```python
from build123d import *

# Parameters (mm, degrees)
EXTRUSION1_DEPTH                  = 3
ESQUISSE2_W                       = 3
ESQUISSE2_H                       = 3
EXTRUSION2_DEPTH                  = 1.2
ESQUISSE3_W                       = 3
ESQUISSE3_H                       = 3
EXTRUSION3_DEPTH                  = 1.2
DIAM_TRE_DU_PER_AGE_4_0_4_1_D     = 4
DIAM_TRE_DU_PER_AGE_4_0_4_1_DEPTH = 3
DIAM_TRE_DU_PER_AGE_4_0_4_1_TIP   = 1.201721238


with BuildPart() as part:
    # Esquisse1 → Extrusion1 (new body, symmetric)
    with BuildSketch(Plane.XY):
        with BuildLine():
            Line((0, 0), (0, 1.5))
            ThreePointArc((0, 1.5), (3.484063784, 6.45860997), (8, 10.5))
            Line((8, 10.5), (30, 10.5))
            Line((30, 10.5), (30, -0.2))
            Line((30, -0.2), (27, -0.2))
            Line((27, -0.2), (27, 3.5))
            Line((27, 3.5), (14, 3.5))
            Line((14, 3.5), (14, 0))
            Line((14, 0), (0, 0))
        make_face()
    extrude(amount=EXTRUSION1_DEPTH, both=True)

    # Esquisse2 → Extrusion2 (add)
    with BuildSketch(Plane(origin=(0, 10.5, 0), x_dir=(1, 0, 0), z_dir=(0, 1, 0))):
        with Locations((28.5, 0)):
            Rectangle(ESQUISSE2_W, ESQUISSE2_H)
    extrude(amount=EXTRUSION2_DEPTH)

    # Esquisse3 → Extrusion3 (add)
    with BuildSketch(Plane.XZ.offset(0.2)):
        with Locations((28.5, 0)):
            Rectangle(ESQUISSE3_W, ESQUISSE3_H)
    extrude(amount=EXTRUSION3_DEPTH)

    # Diamètre du perçage Ø4.0 (4)1
    with Locations(Plane(origin=(30, 0, 0), x_dir=(0, 0, -1), z_dir=(1, 0, 0))):
        with Locations((0, 7)):
            Hole(DIAM_TRE_DU_PER_AGE_4_0_4_1_D / 2, depth=DIAM_TRE_DU_PER_AGE_4_0_4_1_DEPTH)
            with Locations((0, 0, -(DIAM_TRE_DU_PER_AGE_4_0_4_1_DEPTH + DIAM_TRE_DU_PER_AGE_4_0_4_1_TIP / 2))):  # 118° drill point
                Cone(0, DIAM_TRE_DU_PER_AGE_4_0_4_1_D / 2, DIAM_TRE_DU_PER_AGE_4_0_4_1_TIP, mode=Mode.SUBTRACT)


solid = part.part
```
Model file for the job. Use its own axes, mm. A direction names the side the tool comes from. Round coordinates to 2 decimals unless told otherwise and drop trailing zeros. Write each loop counter-clockwise with the first axis right and the second up, starting at its lowest first coordinate (ties: lowest second). Pieces come first, ordered by that corner, then holes. Notation, with made-up numbers: (-3.5, -17.75) - (3.5, -17.75) arc R15 cw to (3.5, -13.75) - close; hole circle Ø8 at (88.5, 87). An arc over 180 degrees is marked (long way). Use CSV: the item, a comma, the result in double quotes. Start each with the question number.
Item 1: Band-saw the part on A-A (z = 2.45). Write the cut outline in (x, y).
Item 2: Band-saw the part on B-B (x = 8.5). Write the cut outline in (y, z), and give its area (3 significant figures).
Item 3: Tool access for faces 1 (the face through (7, 0, 0)), 2 (the face through (28, 11, -1.5)), 3 (the face through (29, -0.2, 2)), 4 (the face through (28, 11, 1.5)), 5 (the face through (28, -1, -1.5)): list every direction of +Z, -Z, +X, -X, +Y, -Y with a clear straight run to the whole face (end or side of a thin tool).
Item 4: Two-plate mould, pull along X, no slides. Class faces 6 (the face through (27, 11, 0)), 7 (the face through (21, 3.5, 0)), 8 (the face through (30, 4, 0)): released by +X, released by -X, zero draft, split by the parting line, or undercut.
Item 5: Band-saw the part on C-C (x = 21.5). Write the cut outline in (y, z).
Item 6: Pin check, flat tips, straight feed: P1, Ø3, axis at y = 5, z = -0.5, coming from the -X side; P2, Ø1, axis at y = 11.5, z = 0.5, coming from the -X side; P3, Ø3, axis at y = 7.5, z = -2, coming from the -X side; P4, Ø1, axis at x = 28, y = -0.5, coming from the +Z side. Stop position of each tip, or through.
Item 7: Drill centre lines: L1, parallel to Y at x = 27.9, z = 0; L2, parallel to Z at x = 28.15, y = 7; L3, parallel to Y at x = 9, z = 0.85. Where is each one in solid material? Low to high. Write a range as [from, to].
Checked values:
1,outline,"(0, 0) - (14, 0) - (14, 3.5) - (27, 3.5) - (27, -0.2) - (30, -0.2) - (30, 10.5) - (8, 10.5) arc R26.6 ccw to (0, 1.5) - close"
2,outline,"(0, -3) - (10.5, -3) - (10.5, 3) - (0, 3) - close"
2,area,"63.0 mm²"
3,face 1,"+Z, -Z, -X, -Y"
3,face 2,"-Z, +X, -X, +Y"
3,face 3,"+Z, +X, -X, -Y"
3,face 4,"+Z, +X, -X, +Y"
3,face 5,"-Z, +X, -X, -Y"
4,face 6,"released by -X"
4,face 7,"undercut"
4,face 8,"released by +X"
5,outline,"(3.5, -3) - (10.5, -3) - (10.5, 3) - (3.5, 3) - close"
6,P1,"stops at x = 1.2"
6,P2,"stops at x = 27"
6,P3,"stops at x = 3.09"
6,P4,"stops at z = 3"
7,L1,"y = [-1.4, 5], [9, 11.7]"
7,L2,"z = [-3, -2], [2, 3]"
7,L3,"y = [0, 10.5]"
